Here's the drawing with two shaded views (mm, measured from the low corner). I have some questions. Coordinates: 2 decimals unless noted, no trailing zeros. Order: outer loops, then holes, each group sorted by start corner. A loop starts at its lowest first (then second) coordinate and runs counter-clockwise, first axis right, second up. Notation, with made-up numbers: (-7, -10.5) - (12, -10.5) arc R13 cw to (12, 8.5) - close; hole circle Ø6 at (-37.5, -14.5). An arc over 180 degrees is marked (long way). Answer as CSV lines item,"result". Start each with the question number.
1. I need wall thicknesses on probe 1 along X at (y, z) = (3.65, 28.5); probe 2 along X at (y, z) = (5.6, 30.5); probe 3 along Z at (x, y) = (83.2, 3.7). Which ranges of each line are inside material? Lowest first, please.
2. I want a section at A-A, the plane y = 3.4. Count the separate pieces of the cut face and the enclosed holes in it, and give its area (3 significant figures).
3. For pin 1 (7 mm diameter, centred on x = 83.2, z = 39.2, fed in from +Y), with a flat end and sliding along its axis, tell me the tip position at first contact or that it passes through.
4. I want a section at C-C, the plane x = 84.7. List the corners of the cut face in (y, z) for me.
5. Thinking about a two-plate mould opening in X: for the marked faces 1 and 2, which applies, released by +X, released by -X, zero draft, split by the parting line, or undercut?
6. I want a section at B-B, the plane z = 29.3. List the corners of the cut face in (x, y) for me, and give its area (3 significant figures).
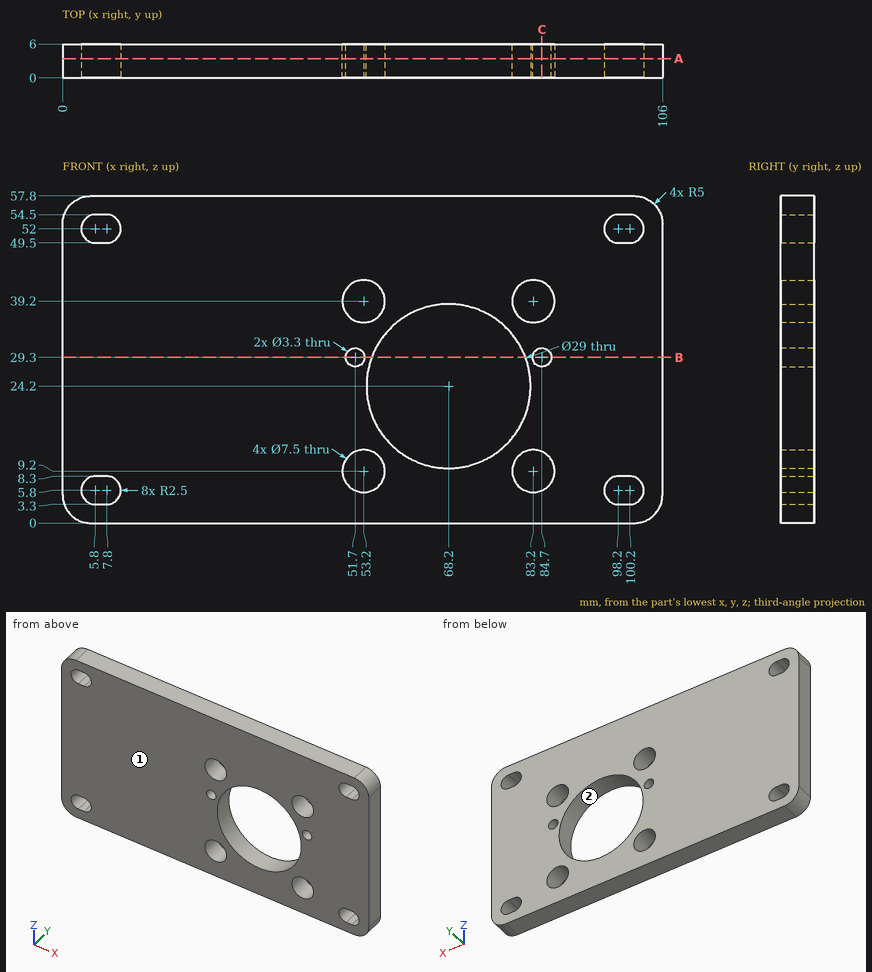
Solved:
1,probe 1,"x = 0 to 50.26, 53.14 to 54.35, 82.05 to 83.26, 86.14 to 106"
1,probe 2,"x = 0 to 50.57, 52.83 to 55.14, 81.26 to 83.57, 85.83 to 106"
1,probe 3,"z = 0 to 5.45, 12.95 to 28.61, 29.99 to 35.45, 42.95 to 57.8"
2,separate pieces,"1"
2,enclosed holes,"11"
2,area,"5,130 mm2"
3,pin 1,"passes through"
4,outline,"(0, 0) - (6, 0) - (6, 5.76) - (0, 5.76) - close; (0, 12.64) - (6, 12.64) - (6, 27.65) - (0, 27.65) - close; (0, 30.95) - (6, 30.95) - (6, 35.76) - (0, 35.76) - close; (0, 42.64) - (6, 42.64) - (6, 57.8) - (0, 57.8) - close"
5,face 1,"zero draft"
5,face 2,"undercut"
6,outline,"(0, 0) - (50.05, 0) - (50.05, 6) - (0, 6) - close; (53.35, 0) - (54.63, 0) - (54.63, 6) - (53.35, 6) - close; (81.77, 0) - (83.05, 0) - (83.05, 6) - (81.77, 6) - close; (86.35, 0) - (106, 0) - (106, 6) - (86.35, 6) - close"
6,area,"434 mm2"
